Design review of the part built by this model. Coordinates are the model's own, in mm. A direction names the side the tool comes from. Give positions to 0.01 mm unless a question says otherwise; leave off trailing zeros. Write each loop counter-clockwise with the first axis right and the second up, starting at its lowest first coordinate (ties: lowest second). Pieces come first, ordered by that corner, then holes. Notation, with made-up numbers: M 8,38 L 30,38 A15 ccw 30,64 Z; hole C 0.25,73 d11. An arc over 180 degrees is marked long. Write each question's results on one line, items separated by ' | '. Start each with the question number.
from build123d import *

# Parameters (mm, degrees)
SKETCH1_W           = 155
SKETCH1_H           = 60
BOSS_EXTRUDE1_DEPTH = 10
SKETCH2_W           = 143
SKETCH2_H           = 20
CUT_EXTRUDE1_DEPTH  = 5
SKETCH3_W           = 10
SKETCH3_H           = 35
BOSS_EXTRUDE2_DEPTH = 78
SKETCH4_W           = 35
SKETCH4_H           = 20
SKETCH4_W_2         = 50
CUT_EXTRUDE2_DEPTH  = 78


with BuildPart() as part:
    # Sketch1 → Boss-Extrude1 (new body)
    with BuildSketch(Plane(origin=(0, 0, 0), x_dir=(1, 0, 0), z_dir=(0, 1, 0))):
        with Locations((77.5, -30)):
            Rectangle(SKETCH1_W, SKETCH1_H)
    extrude(amount=BOSS_EXTRUDE1_DEPTH)

    # Sketch2 → Cut-Extrude1 (cut)
    with BuildSketch(Plane(origin=(0, 10, 0), x_dir=(1, 0, 0), z_dir=(0, 1, 0))):
        with Locations((77.5, -15)):
            Rectangle(SKETCH2_W, SKETCH2_H)
    extrude(amount=-CUT_EXTRUDE1_DEPTH, mode=Mode.SUBTRACT)

    # Sketch3 → Boss-Extrude2 (add)
    with BuildSketch(Plane(origin=(0, 10, 0), x_dir=(1, 0, 0), z_dir=(0, 1, 0))):
        with Locations((5, -42.5)):
            Rectangle(SKETCH3_W, SKETCH3_H)
        with Locations((150, -42.5)):
            Rectangle(SKETCH3_W, SKETCH3_H)
    extrude(amount=BOSS_EXTRUDE2_DEPTH)

    # Sketch4 → Cut-Extrude2 (cut)
    with BuildSketch(Plane(origin=(0, 5, 0), x_dir=(1, 0, 0), z_dir=(0, 1, 0))):
        with Locations((23.5, -15)):
            Rectangle(SKETCH4_W, SKETCH4_H)
        with Locations((124, -15)):
            Rectangle(SKETCH4_W_2, SKETCH4_H)
    extrude(amount=-CUT_EXTRUDE2_DEPTH, mode=Mode.SUBTRACT)


solid = part.part
Q1. We need section B-B on x = 126. Write out the cut boundary in (y, z).
Q2. For faces 1 (the flat face through (77, 10, 3)), 2 (the flat face through (41, 3, 15)), 3 (the flat face through (145, 48, 43)), 4 (the flat face through (0, 43, 44)), 5 (the flat face through (77, 8, 25)), list the 3-axis set-ups (+Z, -Z, +X, -X, +Y, -Y) from which the entire face can be reached by the end or side of a thin tool; tool diameter is ignored.
Q3. The part is to be moulded in two halves that separate along Z. For faces 6 (the flat face through (77, 8, 60)), 7 (the flat face through (155, 43, 44)), 8 (the flat face through (149, 5, 15)), say which applies: pulls with the +Z half, pulls with the -Z half, needs draft (parallel to the pull), parting line crosses it, or undercut.
Q4. We need section C-C on y = 28. Write out the cut boundary in (x, z), and give its area (3 significant figures).
Q5. For pin 1 Ø17.5 at (y, z) = (67, 39) entering from -X; pin 2 Ø8 at (x, z) = (73.5, 29) entering from +Y; pin 3 Ø16 at (x, z) = (65, 16.5) entering from +Y; pin 4 Ø12.5 at (x, z) = (108.5, 11.5) entering from +Y, all flat-tipped, find the tip position at first contact; note any pin that passes through.
Q6. We need section A-A on z = 12.5. Write out the cut boundary in (x, y), and give its area (3 significant figures).
Q7. We need section D-D on z = 47.5. Write out the cut boundary in (x, y).
Q8. Wall thickness on line 1 along X through (y, z) = (8, 23); line 2 along Z through (x, y) = (144, 7); line 3 along X through (y, z) = (25.5, 43): over which ranges is each line inside the solid? List them lowest first. Write a range as from..to.
Answer sheet:
1) outline: M 0,0 L 10,0 L 10,5 L 0,5 Z; M 0,25 L 10,25 L 10,60 L 0,60 Z
2) face 1: -Z, +X, -X, +Y | face 2: +Y, -Y | face 3: +Z, -Z, +Y | face 4: +Z, -Z, -X, +Y, -Y | face 5: +Y
3) face 6: pulls with the +Z half | face 7: needs draft | face 8: undercut
4) outline: M 0,25 L 10,25 L 10,60 L 0,60 Z; M 145,25 L 155,25 L 155,60 L 145,60 Z | area: 700 mm^2
5) pin 1: x = 0 | pin 2: y = 10 | pin 3: y = 5 | pin 4: through
6) outline: M 0,0 L 6,0 L 6,10 L 0,10 Z; M 41,0 L 99,0 L 99,5 L 41,5 Z; M 149,0 L 155,0 L 155,10 L 149,10 Z | area: 410 mm^2
7) outline: M 0,0 L 155,0 L 155,88 L 145,88 L 145,10 L 10,10 L 10,88 L 0,88 Z
8) line 1: 0..6, 149..155 | line 2: 0..5, 25..60 | line 3: 0..10, 145..155
